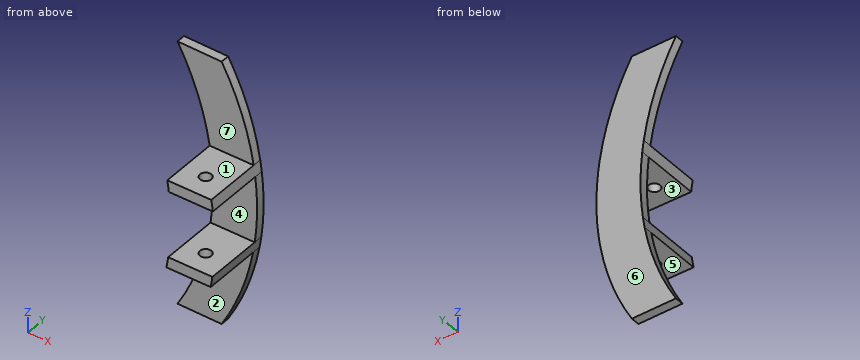
```python
from build123d import *

# Parameters (mm, degrees)
F1_DEPTH = 5.08
F2_DEPTH = 38.1
F4_D     = 6.604


with BuildPart() as f1:
    # F0 (on Front) → F1 (new body)
    with BuildSketch(Plane.XZ):
        with BuildLine():
            Line((-25.397333, -74.747579), (0, -75.115653))
            ThreePointArc((0, -75.115653), (11.223347, -51.049239), (18.098838, -25.4))
            Line((18.098838, -25.4), (-7.363914, -25.4))
            ThreePointArc((-7.363914, -25.4), (-14.238036, -50.856769), (-25.397333, -74.747579))
        make_face()
        with BuildLine():
            Line((-7.363914, -25.4), (18.098838, -25.4))
            ThreePointArc((18.098838, -25.4), (18.623813, -22.230181), (19.081848, -19.05))
            Line((19.081848, -19.05), (-6.365, -19.05))
            ThreePointArc((-6.365, -19.05), (-6.830974, -22.230267), (-7.363914, -25.4))
        make_face()
        with BuildLine():
            Line((-6.365, -19.05), (19.081848, -19.05))
            ThreePointArc((19.081848, -19.05), (20.41381, -0.008572), (19.355084, 19.05))
            Line((19.355084, 19.05), (-5.999007, 19.05))
            ThreePointArc((-5.999007, 19.05), (-4.986636, -0.011483), (-6.365, -19.05))
        make_face()
        with BuildLine():
            Line((-5.999007, 19.05), (19.355084, 19.05))
            ThreePointArc((19.355084, 19.05), (18.943654, 22.229679), (18.465424, 25.4))
            Line((18.465424, 25.4), (-6.872882, 25.4))
            ThreePointArc((-6.872882, 25.4), (-6.402556, 22.229595), (-5.999007, 19.05))
        make_face()
        with BuildLine():
            Line((-6.872882, 25.4), (18.465424, 25.4))
            ThreePointArc((18.465424, 25.4), (11.595818, 52.183193), (0, 77.284347))
            Line((0, 77.284347), (-25.397333, 77.652421))
            ThreePointArc((-25.397333, 77.652421), (-13.739127, 52.37563), (-6.872882, 25.4))
        make_face()
    extrude(amount=F1_DEPTH)

    # F0 (on Front) → F2 (join)
    with BuildSketch(Plane.XZ):
        with BuildLine():
            Line((-5.999007, 19.05), (19.355084, 19.05))
            ThreePointArc((19.355084, 19.05), (18.943654, 22.229679), (18.465424, 25.4))
            Line((18.465424, 25.4), (-6.872882, 25.4))
            ThreePointArc((-6.872882, 25.4), (-6.402556, 22.229595), (-5.999007, 19.05))
        make_face()
        with BuildLine():
            Line((-7.363914, -25.4), (18.098838, -25.4))
            ThreePointArc((18.098838, -25.4), (18.623813, -22.230181), (19.081848, -19.05))
            Line((19.081848, -19.05), (-6.365, -19.05))
            ThreePointArc((-6.365, -19.05), (-6.830974, -22.230267), (-7.363914, -25.4))
        make_face()
    extrude(amount=F2_DEPTH)

    # F4 (through all)
    with Locations(Plane.XY.offset(25.4)):
        with Locations((5.827118, -25.4)):
            Hole(F4_D / 2)


solid = f1.part
```
Can you work these out from the model? Positions are in its coordinate system, mm. Face numbers are marked on the shaded views. A direction names the side the tool comes from. Round coordinates to 2 decimals unless told otherwise and drop trailing zeros. Loops run counter-clockwise (first coordinate to the right, second up) from the corner with the lowest first, then second, coordinate; pieces in that order, holes last. Notation, with made-up numbers: M -4,80.5 L 1,80.5 A23 cw 1,93.5 Z; hole C 37,-38.75 d7. An arc over 180 degrees is marked long. Answer as a JSON object with one key per item and string values. Group by question number.
Q1. Imagine slicing it at A-A, the plane y = -25.4. Please give me the cut outline in (x, z) (3 decimals).
Q2. Imagine slicing it at C-C, the plane x = -18. Please give me the cut outline in (y, z).
Q3. On a 3-axis mill with a long thin cutter (end or side, diameter ignored), from which of +Z, -Z, +X, -X, +Y, -Y can I reach the whole of each face in a straight line? I mean the marked faces 4, 5, 6 and 7. Say none if no direction works.
Q4. Will these pins go through, and if not, where does the flat tip stop? pin 1 (10.5 mm diameter, centred on x = 5.83, y = -25.4, fed in from +Z); pin 2 (12 mm diameter, centred on x = 1.5, z = 59, fed in from +Y); pin 3 (10 mm diameter, centred on x = -7, y = -8, fed in from -Z); pin 4 (4 mm diameter, centred on x = -13, z = 45.5, fed in from -Y).
Q5. Please list where these lines run through material, in increasing order: L1, parallel to Z at x = -5, y = -34; L2, parallel to X at y = -23, z = -23.
Q6. We'd pull the mould along Z, two halves only. Please class the marked faces 1, 2 and 3: +Z half, -Z half, draft (parallel to the pull), parting line (faces both ways), or undercut.
Q7. Imagine slicing it at B-B, the plane y = -31.5. Please give me the cut outline in (x, z) (3 decimals), then the cut area to 3 significant figures.
Q8. Imagine slicing it at D-D, the plane x = -1.5. Please give me the cut outline in (y, z), then the cut area to 3 significant figures.
Findings:
{
 "1": {"outline": "M -7.364,-25.4 L 2.525,-25.4 L 2.525,-19.05 L -6.365,-19.05 A152.402 cw Z; M -6.873,25.4 A152.399 cw -5.999,19.05 L 2.525,19.05 L 2.525,25.4 Z; M 9.129,-25.4 L 18.099,-25.4 A152.403 ccw 19.082,-19.05 L 9.129,-19.05 Z; M 9.129,19.05 L 19.355,19.05 A152.399 ccw 18.465,25.4 L 9.129,25.4 Z"},
 "2": {"outline": "M -5.08,-74.85 L 0,-74.85 L 0,-60.18 L -5.08,-60.18 Z; M -5.08,63.09 L 0,63.09 L 0,77.55 L -5.08,77.55 Z"},
 "3": {"face 4": "+X, -X, -Y", "face 5": "-Z, +X, -X, -Y", "face 6": "+Z, -Z, +X, -X, +Y", "face 7": "+Z, +X, -X, -Y"},
 "4": {"pin 1": "stops at z = 25.4", "pin 2": "stops at y = 0", "pin 3": "stops at z = -75.07", "pin 4": "stops at y = -5.08"},
 "5": {"L1": "z = -25.4 to -19.05, 19.05 to 25.4", "L2": "x = -6.95 to 3.56, 8.09 to 18.5"},
 "6": {"face 1": "+Z half", "face 2": "draft", "face 3": "undercut"},
 "7": {"outline": "M -7.364,-25.4 L 18.099,-25.4 A152.403 ccw 19.082,-19.05 L -6.365,-19.05 A152.402 cw Z; M -6.873,25.4 A152.399 cw -5.999,19.05 L 19.355,19.05 A152.399 ccw 18.465,25.4 Z", "area": "323 mm2"},
 "8": {"outline": "M -38.1,-25.4 L -5.08,-25.4 L -5.08,-75.09 L 0,-75.09 L 0,77.31 L -5.08,77.31 L -5.08,25.4 L -38.1,25.4 L -38.1,19.05 L -5.08,19.05 L -5.08,-19.05 L -38.1,-19.05 Z", "area": "1,190 mm2"}
}
